Can you work these out from the model? Positions are in its coordinate system, mm. Coordinates: 2 decimals unless noted, no trailing zeros. Loops run counter-clockwise (first coordinate to the right, second up) from the corner with the lowest first, then second, coordinate; pieces in that order, holes last.
```python
from build123d import *

# Parameters (mm, degrees)
SKETCH1_W           = 32.1056
SKETCH1_H           = 60.1726
BOSS_EXTRUDE1_DEPTH = 4.2926
SKETCH2_R           = 1.75
SKETCH2_R_2         = 1
CUT_EXTRUDE1_DEPTH  = 5.2926


with BuildPart() as part:
    # Sketch1 → Boss-Extrude1 (new body)
    with BuildSketch(Plane(origin=(0, 0, 0), x_dir=(1, 0, 0), z_dir=(0, 1, 0))):
        with Locations((0, 30.0863)):
            Rectangle(SKETCH1_W, SKETCH1_H)
    extrude(amount=BOSS_EXTRUDE1_DEPTH)

    # Sketch2 → Cut-Extrude1 (cut, through all)
    with BuildSketch(Plane(origin=(0, 4.2926, 0), x_dir=(1, 0, 0), z_dir=(0, 1, 0))):
        with Locations((-9.772224543, 55.4226)):
            Circle(SKETCH2_R)
        with Locations((0.227775457, 55.4226)):
            Circle(SKETCH2_R)
        with Locations((10.227775457, 55.4226)):
            Circle(SKETCH2_R)
        with Locations((-7.272224543, 3.3726)):
            Circle(SKETCH2_R)
        with Locations((-7.272224543, 23.3726)):
            Circle(SKETCH2_R)
        with Locations((7.727775457, 23.3726)):
            Circle(SKETCH2_R)
        with Locations((7.727775457, 3.3726)):
            Circle(SKETCH2_R)
        with Locations((13.977775457, 30.4226)):
            Circle(SKETCH2_R_2)
        with Locations((13.977775457, 37.9226)):
            Circle(SKETCH2_R_2)
        with Locations((-13.522224543, 37.9226)):
            Circle(SKETCH2_R_2)
        with Locations((-13.522224543, 30.4226)):
            Circle(SKETCH2_R_2)
    extrude(amount=-CUT_EXTRUDE1_DEPTH, mode=Mode.SUBTRACT)


solid = part.part
```
Item 1: Suppose I cut it at C-C, the plane x = -7. Please give me the cut outline in (y, z).
Results are:
outline: (0, -60.17) - (4.29, -60.17) - (4.29, -25.1) - (0, -25.1) - close; (0, -21.64) - (4.29, -21.64) - (4.29, -5.1) - (0, -5.1) - close; (0, -1.64) - (4.29, -1.64) - (4.29, 0) - (0, 0) - close
Item 2: We'd pull the mould along X, two halves only. Please class faces 1 (the face through (-5.603, 2.176, -23.898)), 2 (the face through (0, 2, 0)), 3 (the face through (-16.053, 2, -30)): +X half, -X half, draft (parallel to the pull), parting line (faces both ways), or undercut.
Results are:
face 1: undercut
face 2: draft
face 3: -X half
Item 3: I need wall thicknesses on line 1 along Z through (x, y) = (-7, 4.15); line 2 along Z through (x, y) = (-8.5, 1.4); line 3 along X through (y, z) = (3, -30.5). Which ranges of each line are inside material? Lowest first, please.
Results are:
line 1: z = -60.17 to -25.1, -21.64 to -5.1, -1.64 to 0
line 2: z = -60.17 to -56.62, -54.22 to -24.62, -22.13 to -4.62, -2.13 to 0
line 3: x = -16.05 to -14.52, -12.53 to 12.98, 14.97 to 16.05
Item 4: Suppose I cut it at A-A, the plane x = 0.5. Please give me the cut outline in (y, z).
Results are:
outline: (0, -60.17) - (4.29, -60.17) - (4.29, -57.15) - (0, -57.15) - close; (0, -53.69) - (4.29, -53.69) - (4.29, 0) - (0, 0) - close
Item 5: I'm going to push a flat-ended pin straight in: P1, Ø1.5, axis at x = -2, z = -37, coming from the -Y side. Where does the tip first touch, or does it pass through?
Results are:
P1: stops at y = 0
Item 6: Suppose I cut it at B-B, the plane y = 2.95. Count the separate pieces of the cut face and the enclosed holes in it, plus the area to 3 significant figures.
Results are:
separate pieces: 1
enclosed holes: 11
area: 1,850 mm2
